Build history of the part. All positions in model axes, mm. A direction names the side the tool comes from. Give positions to 0.01 mm unless a question says otherwise; leave off trailing zeros. Write each loop counter-clockwise with the first axis right and the second up, starting at its lowest first coordinate (ties: lowest second). Pieces come first, ordered by that corner, then holes. Notation, with made-up numbers: (17, 25) -> (42, 25) arc R19 cw to (42, 29) -> close; hole circle Ø2 at (60, 22.5). An arc over 180 degrees is marked (long way). Put each result on its own line as item: value. Start each with the question number.
Item 1: Tool access for faces 4 (the flat face through (-42, -78, 0)), 5 (the flat face through (-18.529, -77, 13)), 6 (the flat face through (-31, -60.78, 13)): list every direction of +Z, -Z, +X, -X, +Y, -Y with a clear straight run to the whole face (end or side of a thin tool).
Item 2: Slice it at B-B, the plane y = -91.5. List the corners of the cut face in (x, z).
Item 3: Two-plate mould, pull along X, no slides. Class faces 1 (the flat face through (-49.529, -77, 13)), 2 (the flat face through (-11.817, -77, 13)), 3 (the cylindrical face through (1.531, -119.693, 2.465)): pulls with the +X half, pulls with the -X half, needs draft (parallel to the pull), parting line crosses it, or undercut.
Item 4: Slice it at A-A, the plane z = 18.5. List the corners of the cut face in (x, y).
Item 5: Slice it at C-C, the plane x = -20. List the corners of the cut face in (y, z), plus the area to 3 significant figures.
Item 6: Slice it at D-D, the plane y = -79. List the corners of the cut face in (x, z), plus the area to 3 significant figures.
Item 7: Drill centre lines: line 1 along Y through (x, z) = (-24, 12.75); line 2 along Z through (x, y) = (1, -114); line 3 along Y through (x, z) = (-47, 18.25). Where is each one in solid material? Low to high.
Item 8: Flat gauge pins, fed straight in: pin 1 Ø4.5 at (y, z) = (-80, 12.5) entering from -X; pin 2 Ø3 at (x, y) = (-42.53, -121.48) entering from -Z; pin 3 Ø10 at (x, y) = (-73.5, -57.5) entering from +Z; pin 4 Ø4.5 at (x, z) = (-25, 16.5) entering from -Y. Where does each tip first touch, or does it go through?
```python
from build123d import *

# Parameters (mm, degrees)
ESQUISSE1_W        = 108.59
ESQUISSE1_H        = 108.59
ESQUISSE1_R        = 1.8
BOSS_EXTRU_1_DEPTH = 5
ESQUISSE7_W        = 37.712200448
ESQUISSE7_H        = 32.898703175
BOSS_EXTRU_2_DEPTH = 15.5


with BuildPart() as part:
    # Esquisse1 → Boss.-Extru.1 (new body)
    with BuildSketch(Plane(origin=(0, 0, 0), x_dir=(-1, 0, 0), z_dir=(0, 0, 1))):
        with Locations((42.529454852, 77.182817805)):
            Rectangle(ESQUISSE1_W, ESQUISSE1_H)
        with Locations(Location((-1.765545148, 121.477817805, 0), (0, 0, 180))):
            Circle(ESQUISSE1_R, mode=Mode.SUBTRACT)
        with Locations(Location((86.824454852, 121.477817805, 0), (0, 0, 180))):
            Circle(ESQUISSE1_R, mode=Mode.SUBTRACT)
        with Locations(Location((86.824454852, 32.887817805, 0), (0, 0, 180))):
            Circle(ESQUISSE1_R, mode=Mode.SUBTRACT)
        with Locations(Location((-1.765545148, 32.887817805, 0), (0, 0, 180))):
            Circle(ESQUISSE1_R, mode=Mode.SUBTRACT)
        with Locations(Location((42.529454852, 32.887817805, 0), (0, 0, 180))):
            Circle(ESQUISSE1_R, mode=Mode.SUBTRACT)
        with Locations(Location((42.529454852, 121.477817805, 0), (0, 0, 180))):
            Circle(ESQUISSE1_R, mode=Mode.SUBTRACT)
    extrude(amount=BOSS_EXTRU_1_DEPTH)

    # Esquisse7 → Boss.-Extru.2 (add)
    with BuildSketch(Plane.XY.offset(5)):
        with Locations((-30.673354628, -77.229731143)):
            Rectangle(ESQUISSE7_W, ESQUISSE7_H)
        Polygon((-42.529454852, -77.182817805), (-42.529454852, -71.182817805), (-18.529454852, -71.182817805), (-18.529454852, -83.182817805), (-42.529454852, -83.182817805), align=None, mode=Mode.SUBTRACT)
    extrude(amount=BOSS_EXTRU_2_DEPTH)


solid = part.part
```
Values follow:
1. face 4: -Z, +X, -X, +Y, -Y
1. face 5: +Z
1. face 6: +Z, +X, -X, +Y
2. outline: (-96.82, 0) -> (11.77, 0) -> (11.77, 5) -> (-11.82, 5) -> (-11.82, 20.5) -> (-49.53, 20.5) -> (-49.53, 5) -> (-96.82, 5) -> close
3. face 1: pulls with the -X half
3. face 2: pulls with the +X half
3. face 3: undercut
4. outline: (-49.53, -93.68) -> (-11.82, -93.68) -> (-11.82, -60.78) -> (-49.53, -60.78) -> close; hole (-42.53, -83.18) -> (-18.53, -83.18) -> (-18.53, -71.18) -> (-42.53, -71.18) -> close
5. outline: (-131.48, 0) -> (-22.89, 0) -> (-22.89, 5) -> (-60.78, 5) -> (-60.78, 20.5) -> (-71.18, 20.5) -> (-71.18, 5) -> (-83.18, 5) -> (-83.18, 20.5) -> (-93.68, 20.5) -> (-93.68, 5) -> (-131.48, 5) -> close
5. area: 867 mm2
6. outline: (-96.82, 0) -> (11.77, 0) -> (11.77, 5) -> (-11.82, 5) -> (-11.82, 20.5) -> (-18.53, 20.5) -> (-18.53, 5) -> (-42.53, 5) -> (-42.53, 20.5) -> (-49.53, 20.5) -> (-49.53, 5) -> (-96.82, 5) -> close
6. area: 755 mm2
7. line 1: -93.68 to -83.18, -71.18 to -60.78
7. line 2: 0 to 5
7. line 3: -93.68 to -60.78
8. pin 1: x = -49.53
8. pin 2: through
8. pin 3: z = 5
8. pin 4: y = -93.68
